The figure shows three views and two pictorial views of one solid part (mm, origin at its lowest corner). Answer the questions. A direction names the side the tool comes from. Give positions to 0.01 mm unless a question says otherwise; leave off trailing zeros. Order: outer loops, then holes, each group sorted by start corner. A loop starts at its lowest first (then second) coordinate and runs counter-clockwise, first axis right, second up. Notation, with made-up numbers: (8.5, 78.25) - (34.5, 78.25) arc R20 cw to (34.5, 116.25) - close; hole circle Ø3 at (87.25, 86). An arc over 180 degrees is marked (long way). Return JSON: item names as keys, results as strings. Group by question number.
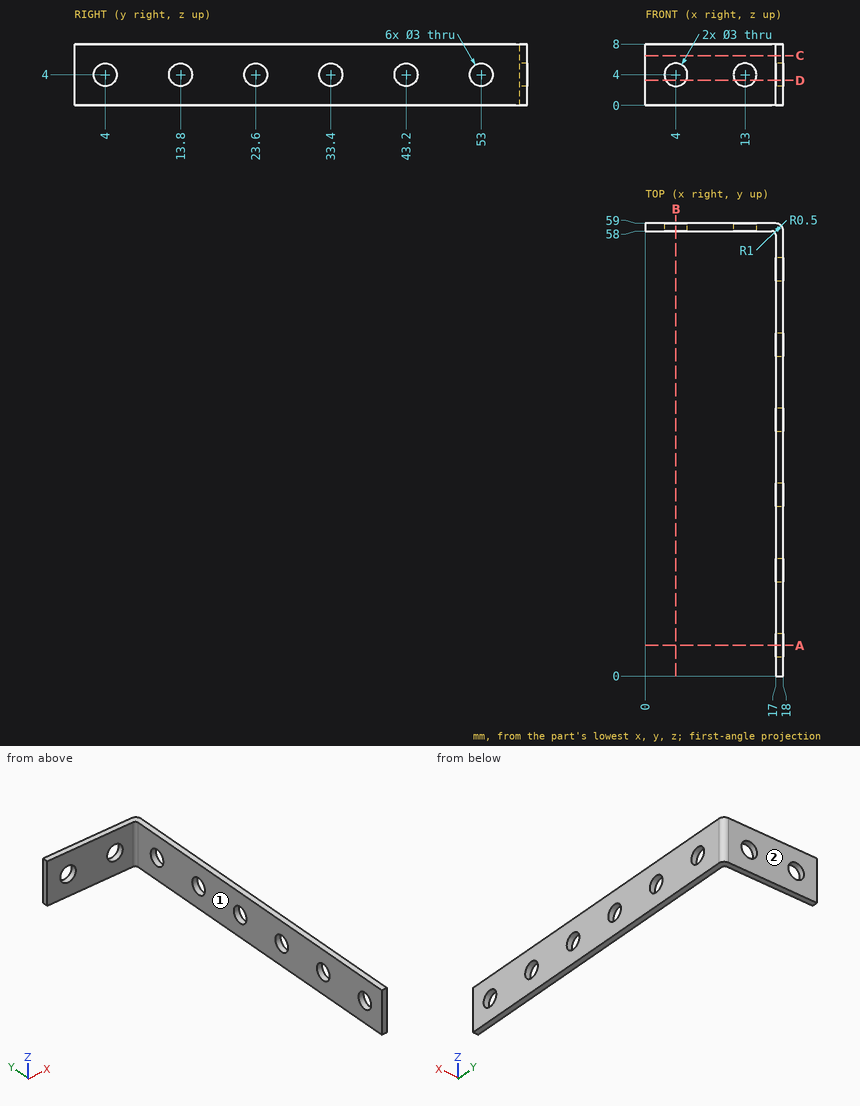
1. The part is cut by section C-C (z = 6.5). Give the vertices of the cut face in (x, y).
2. Each of these flat-tipped pins is pushed along its axis until it touches: pin 1 (2.5 mm diameter, centred on x = 13, z = 4, fed in from -Y); pin 2 (1.5 mm diameter, centred on y = 16.5, z = 4, fed in from -X); pin 3 (1.5 mm diameter, centred on x = 7, z = 3.5, fed in from -Y). Where does it stop, or does it pass through?
3. The part is cut by section D-D (z = 3.25). State how many separate pieces and enclosed holes the cut face has, and give its area (3 significant figures).
4. Consider probe 1 along Z at (x, y) = (17.4, 53); probe 2 along Y at (x, z) = (9.5, 3.5); probe 3 along X at (y, z) = (35, 7.5). Determine where each line is inside the solid, lowest interval first. Write a range as from..to.
5. A tool of negligible diameter and unlimited length cuts with its end or side. For the marked faces 1 and 2, from which of +Z, -Z, +X, -X, +Y, -Y can it reach the whole face along a straight path? Write none if from no direction.
6. The part is cut by section B-B (x = 4). Give the vertices of the cut face in (y, z).
7. The part is cut by section A-A (y = 4). Give the vertices of the cut face in (x, z), and give its area (3 significant figures).
Answers:
{
 "1": {"outline": "(0, 58) - (16.5, 58) arc R0.5 cw to (17, 57.5) - (17, 0) - (18, 0) - (18, 58) arc R1 ccw to (17, 59) - (0, 59) - close"},
 "2": {"pin 1": "passes through", "pin 2": "stops at x = 17", "pin 3": "stops at y = 58"},
 "3": {"separate pieces": "9", "enclosed holes": "0", "area": "55.1 mm^2"},
 "4": {"probe 1": "z = 0..2.5, 5.5..8", "probe 2": "y = 58..59", "probe 3": "x = 17..18"},
 "5": {"face 1": "+Z, -Z, -X, -Y", "face 2": "+Z, -Z, +X, -X, +Y"},
 "6": {"outline": "(58, 0) - (59, 0) - (59, 2.5) - (58, 2.5) - close; (58, 5.5) - (59, 5.5) - (59, 8) - (58, 8) - close"},
 "7": {"outline": "(17, 0) - (18, 0) - (18, 2.5) - (17, 2.5) - close; (17, 5.5) - (18, 5.5) - (18, 8) - (17, 8) - close", "area": "5.00 mm^2"}
}
